Here's how the part is built. I have some questions about the finished solid (model axes, mm). Round coordinates to 2 decimals unless told otherwise and drop trailing zeros. Write each loop counter-clockwise with the first axis right and the second up, starting at its lowest first coordinate (ties: lowest second). Pieces come first, ordered by that corner, then holes. Notation, with made-up numbers: (-17, 8) -> (-7, 8) arc R28 cw to (-7, 35) -> close; hole circle Ø8 at (-2, 36.25). An arc over 180 degrees is marked (long way). Put each result on its own line as item: value. Start each with the question number.
1) We'd pull the mould along X, two halves only. Please class faces 1 (the flat face through (-1, 1, 0)), 2 (the cylindrical face through (-69.245, 41.374, -0.798)), 3 (the cylindrical face through (-72.7, -39.38, -0.8)), 4 (the cylindrical face through (84.795, 26.703, -0.776)): released by +X, released by -X, zero draft, split by the parting line, or undercut.
2) I want a section at B-B, the plane y = -82.55. List the corners of the cut face in (x, z) for me, then the cut area to 3 significant figures.
3) I want a section at D-D, the plane y = 66. List the corners of the cut face in (x, z) for me, then the cut area to 3 significant figures.
4) I want a section at A-A, the plane x = 0. List the corners of the cut face in (y, z) for me, then the cut area to 3 significant figures.
5) I want a section at C-C, the plane z = -0.35. Give the number of separate pieces and of enclosed holes in the cut face, then the cut area to 3 significant figures.
6) Will this pin go through, and if not, where does the flat tip stop? P1, Ø5, axis at x = -71.49, y = -41.27, coming from the +Z side.
7) If I drill on line 1 along Y through (x, z) = (0, -1.15); line 2 along Y through (x, z) = (-69.5, -1.3); line 3 along X through (y, z) = (52, -0.5), over which ranges is the centre line in solid material (lowest first)? Write a range as [from, to].
from build123d import *

# Parameters (mm, degrees)
F0_R     = 88.9
F1_DEPTH = 1.5748
F3_D     = 4.4958
F5_D     = 4.4958


with BuildPart() as f1:
    # F0 (on Top) → F1 (new body)
    with BuildSketch(Plane.XY):
        Circle(F0_R)
    extrude(amount=-F1_DEPTH)

    # F3 (through all)
    with Locations(Plane.XY):
        with Locations((0, 82.55), (-71.490402, -41.274992), (71.490395, -41.275004)):
            Hole(F3_D / 2)

    # F5 (through all)
    with Locations(Plane.XY):
        with Locations((0, -82.55), (71.490397, 41.275), (-71.490397, 41.275)):
            Hole(F5_D / 2)


solid = f1.part
Findings:
1. face 1: zero draft
1. face 2: undercut
1. face 3: undercut
1. face 4: split by the parting line
2. outline: (-33, -1.57) -> (-2.25, -1.57) -> (-2.25, 0) -> (-33, 0) -> close; (2.25, -1.57) -> (33, -1.57) -> (33, 0) -> (2.25, 0) -> close
2. area: 96.8 mm2
3. outline: (-59.56, -1.57) -> (59.56, -1.57) -> (59.56, 0) -> (-59.56, 0) -> close
3. area: 188 mm2
4. outline: (-88.9, -1.57) -> (-84.8, -1.57) -> (-84.8, 0) -> (-88.9, 0) -> close; (-80.3, -1.57) -> (80.3, -1.57) -> (80.3, 0) -> (-80.3, 0) -> close; (84.8, -1.57) -> (88.9, -1.57) -> (88.9, 0) -> (84.8, 0) -> close
4. area: 266 mm2
5. separate pieces: 1
5. enclosed holes: 6
5. area: 24,700 mm2
6. P1: stops at z = 0
7. line 1: y = [-88.9, -84.8], [-80.3, 80.3], [84.8, 88.9]
7. line 2: y = [-55.43, -42.32], [-40.23, 40.23], [42.32, 55.43]
7. line 3: x = [-72.11, 72.11]
